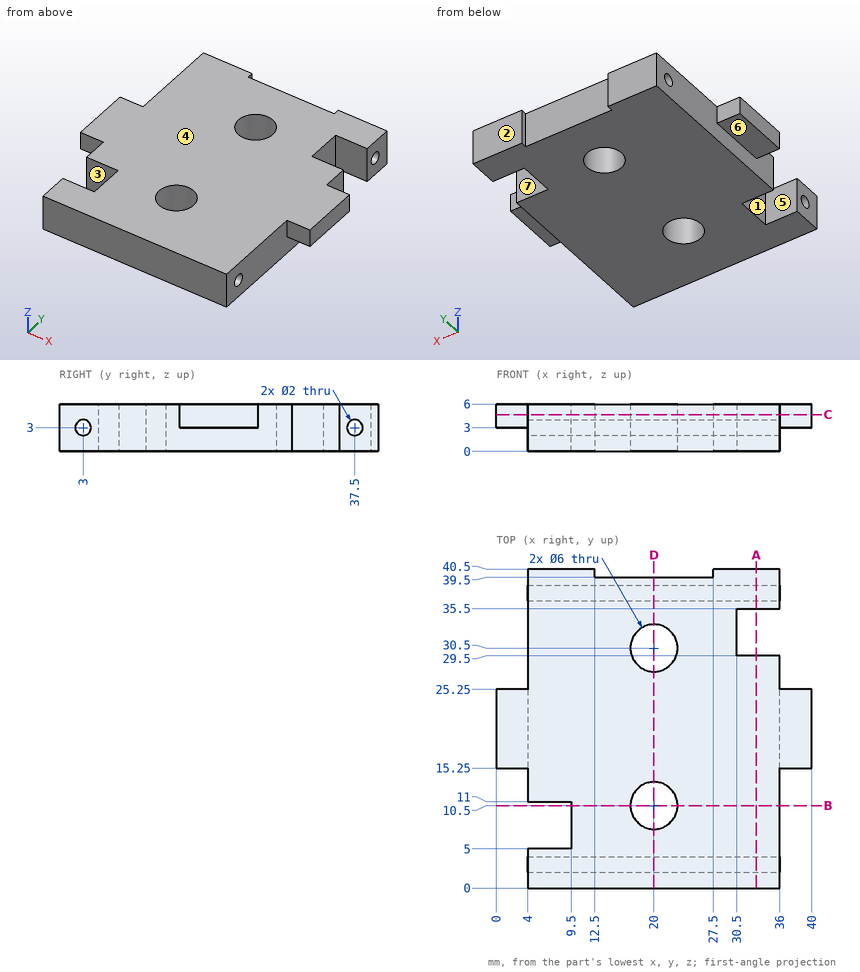
Print and shaded views of the part. All mm, measured from the part's lowest x, y and z. A direction names the side the tool comes from. Round coordinates to 2 decimals unless told otherwise and drop trailing zeros. Order: outer loops, then holes, each group sorted by start corner. A loop starts at its lowest first (then second) coordinate and runs counter-clockwise, first axis right, second up.
Q1. Wall check: L1, parallel to Y at x = 20, z = 4.8; L2, parallel to Y at x = 25, z = 3; L3, parallel to Y at x = 34.5, z = 5.2. Give the ranges that are in metal, low to high.
Q2. Drop flat-ended pins along their axis: pin 1 (2 mm diameter, centred on y = 10, z = 3, fed in from +X); pin 2 (3 mm diameter, centred on x = 1.5, y = 19, fed in from -Z); pin 3 (1.1 mm diameter, centred on y = 40, z = 1.5, fed in from -X). Give the stop position or say it passes through.
Q3. Slice it at C-C (z = 4.65). Write the cut outline in (x, y).
Q4. Which spindle directions (+Z, -Z, +X, -X, +Y, -Y) get a long thin tool onto all of the face, cutting with end or side? Do the marked faces 5, 6 and 7. Say none if no direction does.
Q5. Slice it at B-B (y = 10.5). Write the cut outline in (x, z).
Q6. Slice it at A-A (x = 33). Write the cut outline in (y, z).
Q7. Slice it at D-D (x = 20). Write the cut outline in (y, z).
Q8. Two-plate mould, pull along Y, no slides. Class the marked faces 1, 2, 3 and 4: pulls with the +Y half, pulls with the -Y half, needs draft (parallel to the pull), parting line crosses it, or undercut.
Results below:
1. L1: y = 0 to 7.5, 13.5 to 27.5, 33.5 to 39.5
1. L2: y = 0 to 2, 4 to 36.5, 38.5 to 39.5
1. L3: y = 0 to 29.5, 35.5 to 40.5
2. pin 1: stops at x = 36
2. pin 2: stops at z = 3
2. pin 3: stops at x = 4
3. outline: (0, 15.25) - (4, 15.25) - (4, 11) - (9.5, 11) - (9.5, 5) - (4, 5) - (4, 0) - (36, 0) - (36, 15.25) - (40, 15.25) - (40, 25.25) - (36, 25.25) - (36, 29.5) - (30.5, 29.5) - (30.5, 35.5) - (36, 35.5) - (36, 40.5) - (27.5, 40.5) - (27.5, 39.5) - (12.5, 39.5) - (12.5, 40.5) - (4, 40.5) - (4, 25.25) - (0, 25.25) - close; hole circle Ø6 at (20, 10.5); hole circle Ø6 at (20, 30.5)
4. face 5: +Z, -Z, -X
4. face 6: -Z, -X, +Y, -Y
4. face 7: +Z, -Z, +X
5. outline: (9.5, 0) - (17, 0) - (17, 6) - (9.5, 6) - close; (23, 0) - (36, 0) - (36, 6) - (23, 6) - close
6. outline: (0, 0) - (29.5, 0) - (29.5, 6) - (0, 6) - close; (35.5, 0) - (40.5, 0) - (40.5, 6) - (35.5, 6) - close; hole circle Ø2 at (3, 3); hole circle Ø2 at (37.5, 3)
7. outline: (0, 0) - (7.5, 0) - (7.5, 6) - (0, 6) - close; (13.5, 0) - (27.5, 0) - (27.5, 6) - (13.5, 6) - close; (33.5, 0) - (39.5, 0) - (39.5, 6) - (33.5, 6) - close; hole circle Ø2 at (3, 3); hole circle Ø2 at (37.5, 3)
8. face 1: undercut
8. face 2: pulls with the +Y half
8. face 3: undercut
8. face 4: needs draft
